Source: three-view drawing plus pictorial views. Frame: mm from the lowest corner of the part. A direction names the side the tool comes from. Give positions to 0.01 mm unless a question says otherwise; leave off trailing zeros. Write each loop counter-clockwise with the first axis right and the second up, starting at its lowest first coordinate (ties: lowest second). Pieces come first, ordered by that corner, then holes. Notation, with made-up numbers: (49, 76.25) -> (90, 76.25) arc R17 cw to (90, 80.25) -> close; hole circle Ø2 at (27, 12). An arc over 180 degrees is marked (long way). Answer in a Markdown table with one row per item. Add a question column.
Item 1: Section query A-A on y = 355.6. Output: boundary loops of the cut face in (x, z) (1 decimal).
Item 2: Section query D-D on x = 1641. Output: boundary loops of the cut face in (y, z) (1 decimal), plus the area to 3 significant figures.
Item 3: Section query C-C on y = 879.5. Output: boundary loops of the cut face in (x, z).
Item 4: Material intervals for probe 1 along Y at (x, z) = (838.5, 92) (1 decimal); probe 2 along Y at (x, z) = (843.5, 138); probe 3 along Y at (x, z) = (389.5, 80) (1 decimal), sorted ascending. Write a range as from..to.
Item 5: First-contact query: P1, Ø8, axis at x = 653, z = 70, coming from the +Y side (1 decimal); P2, Ø5, axis at x = 637, z = 44.5, coming from the +Y side; P3, Ø6, axis at y = 1574.5, z = 50, coming from the +X side. Flat tips, straight axial feed; report the tip coordinate or a pass-through.
Item 6: Section query B-B on x = 1235. Output: boundary loops of the cut face in (y, z), plus the area to 3 significant figures.
Item 7: Access query for the marked faces 4, 5 and 6. Directions: +Z, -Z, +X, -X, +Y, -Y. A direction counts if a zero-diameter tool reaches every point of the face in a straight line with its end or side. Return the directions, or none.
Item 8: Draft query along X for the marked faces 1, 2 and 3. Return one class per face: +X half, -X half, draft (parallel to the pull), parting line (faces both ways), or undercut.
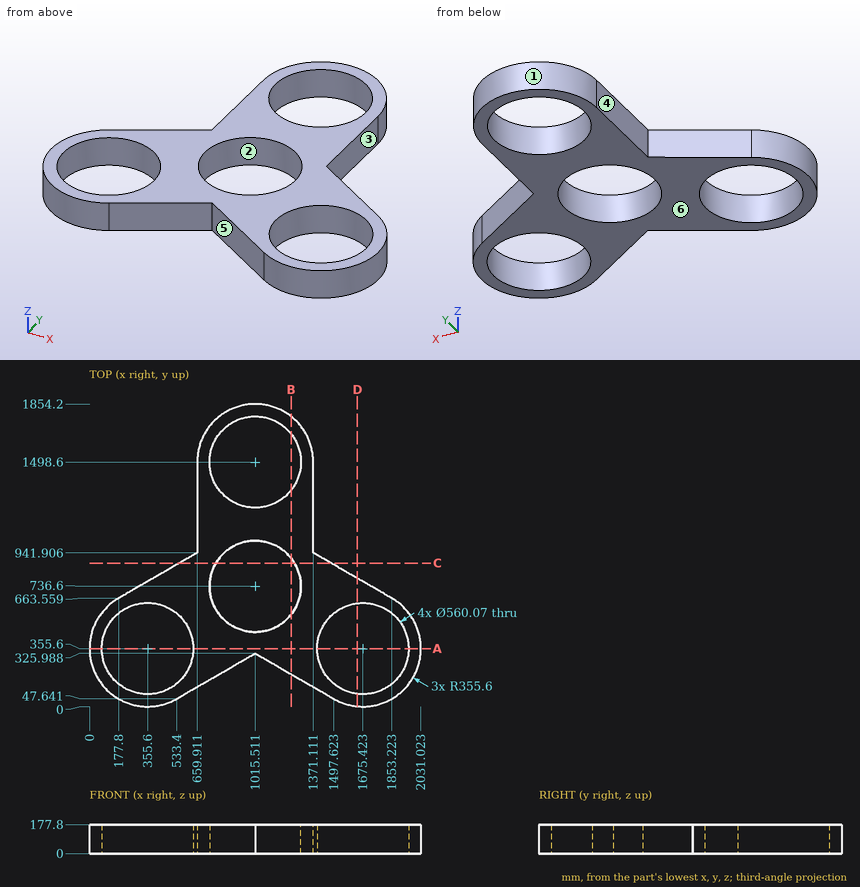
Findings below:
| question | item | result |
|---|---|---|
| 1 | outline | (0, 0) -> (75.6, 0) -> (75.6, 177.8) -> (0, 177.8) -> close; (635.6, 0) -> (1395.4, 0) -> (1395.4, 177.8) -> (635.6, 177.8) -> close; (1955.5, 0) -> (2031, 0) -> (2031, 177.8) -> (1955.5, 177.8) -> close |
| 2 | outline | (1.7, 0) -> (77.7, 0) -> (77.7, 177.8) -> (1.7, 177.8) -> close; (633.5, 0) -> (786.1, 0) -> (786.1, 177.8) -> (633.5, 177.8) -> close |
| 2 | area | 40,600 mm^2 |
| 3 | outline | (551.82, 0) -> (774.68, 0) -> (774.68, 177.8) -> (551.82, 177.8) -> close; (1256.34, 0) -> (1479.2, 0) -> (1479.2, 177.8) -> (1256.34, 177.8) -> close |
| 4 | probe 1 | y = 223.8..519.6, 953.6..1281.6, 1715.6..1807 |
| 4 | probe 2 | y = 226.68..515.62, 957.58..1277.62, 1719.58..1809.83 |
| 4 | probe 3 | y = 1.6..77.6, 633.6..785.8 |
| 5 | P1 | stops at y = 940.2 |
| 5 | P2 | stops at y = 930.12 |
| 5 | P3 | stops at x = 1363.56 |
| 6 | outline | (199.27, 0) -> (562.69, 0) -> (562.69, 177.8) -> (199.27, 177.8) -> close; (910.51, 0) -> (1324.69, 0) -> (1324.69, 177.8) -> (910.51, 177.8) -> close; (1672.51, 0) -> (1778.38, 0) -> (1778.38, 177.8) -> (1672.51, 177.8) -> close |
| 6 | area | 157,000 mm^2 |
| 7 | face 4 | +Z, -Z, -X, +Y |
| 7 | face 5 | +Z, -Z, -Y |
| 7 | face 6 | -Z, +X, -X, +Y, -Y |
| 8 | face 1 | parting line |
| 8 | face 2 | undercut |
| 8 | face 3 | +X half |
